from build123d import *
from OCP.BRepFilletAPI import BRepFilletAPI_MakeChamfer

# Parameters (mm, degrees)
SKETCH_1_W          = 26
SKETCH_1_H          = 56
EXTRUDE_1_DEPTH     = 10.61
SKETCH_2_R          = 1.65
SKETCH_2_W          = 20.7
SKETCH_2_H          = 41.3
CUT_EXTRUDE_1_DEPTH = 33.643101875
SKETCH_3_W          = 2.5
SKETCH_3_H          = 56
CUT_EXTRUDE_2_DEPTH = 2.5
SKETCH_4_W          = 23.2
SKETCH_4_H          = 2.8
SKETCH_4_W_2        = 2.5
SKETCH_4_H_2        = 3.1
EXTRUDE_2_DEPTH     = 7.35
SKETCH_5_W          = 23.2
SKETCH_5_H          = 8.527384077
EXTRUDE_5_DEPTH     = 1.2
SKETCH_6_R          = 1.65
CUT_EXTRUDE_3_DEPTH = 36.975270673
CHAMFER_1_SIZE      = 4.5
CHAMFER_1_SIZE2     = 2.598076211
CHAMFER_2_SIZE      = 1
CHAMFER_3_SIZE      = 6
CHAMFER_6_SIZE      = 3.6


with BuildPart() as part:
    # 草图1 → 凸台-拉伸1 (new body)
    with BuildSketch(Plane(origin=(0, 0, 0), x_dir=(1, 0, 0), z_dir=(0, 1, 0))):
        Rectangle(SKETCH_1_W, SKETCH_1_H)
    extrude(amount=EXTRUDE_1_DEPTH)

    # 草图2 → 切除-拉伸1 (cut, through all)
    with BuildSketch(Plane(origin=(0, 10.61, 0), x_dir=(1, 0, 0), z_dir=(0, 1, 0))):
        with Locations(Location((-7.9, 24.25, 0), (0, 0, 270))):
            Circle(SKETCH_2_R)
        with Locations(Location((2.6, 24.25, 0), (0, 0, 90))):
            Circle(SKETCH_2_R)
        with Locations(Location((2.6, -24.25, 0), (0, 0, 270))):
            Circle(SKETCH_2_R)
        with Locations(Location((-7.9, -24.25, 0), (0, 0, 90))):
            Circle(SKETCH_2_R)
        with Locations((-2.65, 0)):
            Rectangle(SKETCH_2_W, SKETCH_2_H)
    extrude(amount=-CUT_EXTRUDE_1_DEPTH, mode=Mode.SUBTRACT)

    # 草图3 → 切除-拉伸2 (cut)
    with BuildSketch(Plane(origin=(0, 10.61, 0), x_dir=(1, 0, 0), z_dir=(0, 1, 0))):
        with Locations((-2.65, 0)):
            Rectangle(SKETCH_3_W, SKETCH_3_H)
    extrude(amount=-CUT_EXTRUDE_2_DEPTH, mode=Mode.SUBTRACT)

    # 草图4 → 凸台-拉伸2 (add)
    with BuildSketch(Plane.XY.offset(-20.65)):
        with Locations((-1.4, 15.11)):
            Rectangle(SKETCH_4_W, SKETCH_4_H)
        with Locations((8.95, 12.16)):
            Rectangle(SKETCH_4_W_2, SKETCH_4_H_2)
    extrude_2 = extrude(amount=-EXTRUDE_2_DEPTH)

    # 草图5 → 凸台-拉伸5 (add)
    with BuildSketch(Plane(origin=(0, 0, -28), x_dir=(-1, 0, 0), z_dir=(0, 0, -1))):
        with Locations((1.4, 12.246307962)):
            Rectangle(SKETCH_5_W, SKETCH_5_H)
    extrude_5 = extrude(amount=EXTRUDE_5_DEPTH)

    # 草图6 → 切除-拉伸3 (cut, through all)
    with BuildSketch(Plane(origin=(0, 16.51, 0), x_dir=(1, 0, 0), z_dir=(0, 1, 0))):
        with Locations(Location((2.6, 24.25, 0), (0, 0, 90))):
            Circle(SKETCH_6_R)
        with Locations(Location((-7.9, 24.25, 0), (0, 0, 270))):
            Circle(SKETCH_6_R)
    cut_extrude_3 = extrude(amount=-CUT_EXTRUDE_3_DEPTH, mode=Mode.SUBTRACT)

    # 镜向2: 凸台-拉伸2, 凸台-拉伸5, 切除-拉伸3 across plane
    add(extrude_2.mirror(Plane.XY))
    add(extrude_5.mirror(Plane.XY))
    add(cut_extrude_3.mirror(Plane.XY), mode=Mode.SUBTRACT)

    # 倒角1: one chamfer whose edges measure the first distance from different faces: ONE call of the kernel's chamfer builder (chamfer() names one face for all edges)
    chamfer_1_edges_1 = [part.edges().sort_by_distance(p)[0] for p in [
        (10.2, 10.61, 24.325),
    ]]
    chamfer_1_side_1 = [part.faces().sort_by_distance(p)[0] for p in [
        (10.2, 13.309190963, 25.141179594),
    ]]
    chamfer_1_edges_2 = [part.edges().sort_by_distance(p)[0] for p in [
        (10.2, 10.61, -24.325),
    ]]
    chamfer_1_side_2 = [part.faces().sort_by_distance(p)[0] for p in [
        (10.2, 13.309190963, -25.141179594),
    ]]
    chamfer_1 = BRepFilletAPI_MakeChamfer(part.part.solid().wrapped)
    for e in chamfer_1_edges_1:
        chamfer_1.Add(CHAMFER_1_SIZE, CHAMFER_1_SIZE2, e.wrapped, chamfer_1_side_1[0].wrapped)  # the first distance lies on this face
    for e in chamfer_1_edges_2:
        chamfer_1.Add(CHAMFER_1_SIZE, CHAMFER_1_SIZE2, e.wrapped, chamfer_1_side_2[0].wrapped)  # the first distance lies on this face
    add(Compound.cast(chamfer_1.Shape()), mode=Mode.REPLACE)

    # 倒角2
    chamfer_2_edges = [part.edges().sort_by_distance(p)[0] for p in [
        (-13, 3.991307961, -28),
        (-1.4, 7.982615923, -28),
        (-13, 7.982615923, -28.6),
        (10.2, 16.51, 24.925),
        (-13, 15.11, 20.65),
        (-13, 3.991307961, 28),
        (-1.4, 7.982615923, 28),
        (-13, 7.982615923, 28.6),
        (-13, 5.305, 20.65),
        (-13, 5.305, -20.65),
        (10.2, 16.51, -24.925),
        (-13, 15.11, -20.65),
    ]]
    chamfer(chamfer_2_edges, length=CHAMFER_2_SIZE)

    # 倒角3
    chamfer_3_edges = [part.edges().sort_by_distance(p)[0] for p in [
        (13, 5.305, 28),
        (13, 5.305, -28),
    ]]
    chamfer(chamfer_3_edges, length=CHAMFER_3_SIZE)

    # 倒角6
    chamfer_6_edges = [part.edges().sort_by_distance(p)[0] for p in [
        (10.2, 11.746307961, 29.2),
        (10.2, 11.746307961, -29.2),
    ]]
    chamfer(chamfer_6_edges, length=CHAMFER_6_SIZE)


solid = part.part
The model under review builds one solid part; all positions refer to its coordinate system, in mm. A direction names the side the tool comes from. Give positions to 0.01 mm unless a question says otherwise; leave off trailing zeros. Write each loop counter-clockwise with the first axis right and the second up, starting at its lowest first coordinate (ties: lowest second). Pieces come first, ordered by that corner, then holes.
1. Add section D-D, the plane y = 12.5. Write out the cut boundary in (x, z), plus the area to 3 significant figures.
2. Tool access review of faces 1 (the flat face through (-3, 8.11, -24)), 2 (the flat face through (-2, 5, 20.65)), 3 (the flat face through (-10, 10.61, 25)), 4 (the flat face through (11, 6, -24)): name each direction out of +Z, -Z, +X, -X, +Y, -Y from which nothing blocks a thin tool from reaching the whole face with its end or side.
3. Add section C-C, the plane z = -24.25. Count the separate pieces of the cut face and the enclosed holes in it, plus the area to 3 significant figures.
4. Add section A-A, the plane x = 0.25. Write out the cut boundary in (y, z), plus the area to 3 significant figures.
5. Add section B-B, the plane y = 1. Write out the cut boundary in (x, z), plus the area to 3 significant figures.
6. Wall thickness on L1, parallel to X at y = 14.4, z = -24.25; L2, parallel to Z at x = 6.25, y = 3.5; L3, parallel to Z at x = -4.75, y = 14: over which ranges is each line inside the solid? List them lowest first.
7. Draft analysis for pull direction X (two halves, no side actions). For faces 5 (the flat face through (-12.51, 5.38, 21.16)), 6 (the flat face through (9.69, 16.02, 23.58)), 7 (the flat face through (-1.4, 9, -24)), state which applies: +X half, -X half, draft (parallel to the pull), parting line (faces both ways), or undercut.
8. For P1, Ø6, axis at x = 10.5, z = 4, coming from the +Y side; P2, Ø2, axis at y = 9.5, z = 24, coming from the +X side; P3, Ø3, axis at y = 3, z = 5, coming from the -X side, all flat-tipped, find the tip position at first contact; note any pin that passes through.
Worked answers:
1. outline: (-13, -29.2) - (6.6, -29.2) - (10.2, -25.6) - (10.2, -24.8) - (11.71, -23.29) - (11.71, -20.65) - (7.7, -20.65) - (7.7, -28) - (-13, -28) - close; (-13, 28) - (7.7, 28) - (7.7, 20.65) - (11.71, 20.65) - (11.71, 23.29) - (10.2, 24.8) - (10.2, 25.6) - (6.6, 29.2) - (-13, 29.2) - close
1. area: 89.7 mm2
2. face 1: none
2. face 2: -X, +Y, -Y
2. face 3: -X
2. face 4: -Z, +X, -Y
3. separate pieces: 5
3. enclosed holes: 0
3. area: 232 mm2
4. outline: (0, -28) - (6.98, -28) - (7.98, -29) - (7.98, -29.2) - (16.51, -29.2) - (16.51, -20.65) - (13.71, -20.65) - (13.71, -28) - (10.61, -28) - (10.61, -20.65) - (0, -20.65) - close; (0, 20.65) - (10.61, 20.65) - (10.61, 28) - (13.71, 28) - (13.71, 20.65) - (16.51, 20.65) - (16.51, 29.2) - (7.98, 29.2) - (7.98, 29) - (6.98, 28) - (0, 28) - close
4. area: 219 mm2
5. outline: (-13, -27) - (-12, -28) - (7, -28) - (13, -22) - (13, 22) - (7, 28) - (-12, 28) - (-13, 27) - (-13, 21.65) - (-12, 20.65) - (7.7, 20.65) - (7.7, -20.65) - (-12, -20.65) - (-13, -21.65) - close; hole circle Ø3.3 at (-7.9, -24.25); hole circle Ø3.3 at (-7.9, 24.25); hole circle Ø3.3 at (2.6, -24.25); hole circle Ø3.3 at (2.6, 24.25)
5. area: 529 mm2
6. L1: x = -13 to -9.55, -6.25 to 0.95, 4.25 to 10.61
6. L2: z = -28 to -20.65, 20.65 to 28
6. L3: z = -29.2 to -20.65, 20.65 to 29.2
7. face 5: -X half
7. face 6: +X half
7. face 7: undercut
8. P1: stops at y = 10.61
8. P2: stops at x = 12
8. P3: stops at x = 7.7
